Verification items for this drawing (mm, ordinates from the low corner). A direction names the side the tool comes from. Coordinates: 2 decimals unless noted, no trailing zeros. Write each loop counter-clockwise with the first axis right and the second up, starting at its lowest first coordinate (ties: lowest second). Pieces come first, ordered by that corner, then holes. Notation, with made-up numbers: (-30.75, 14) -> (12.25, 14) arc R20 cw to (12.25, 49) -> close; hole circle Ø9 at (29, 80). An arc over 180 degrees is marked (long way). One line per question, with ' | ' between items.
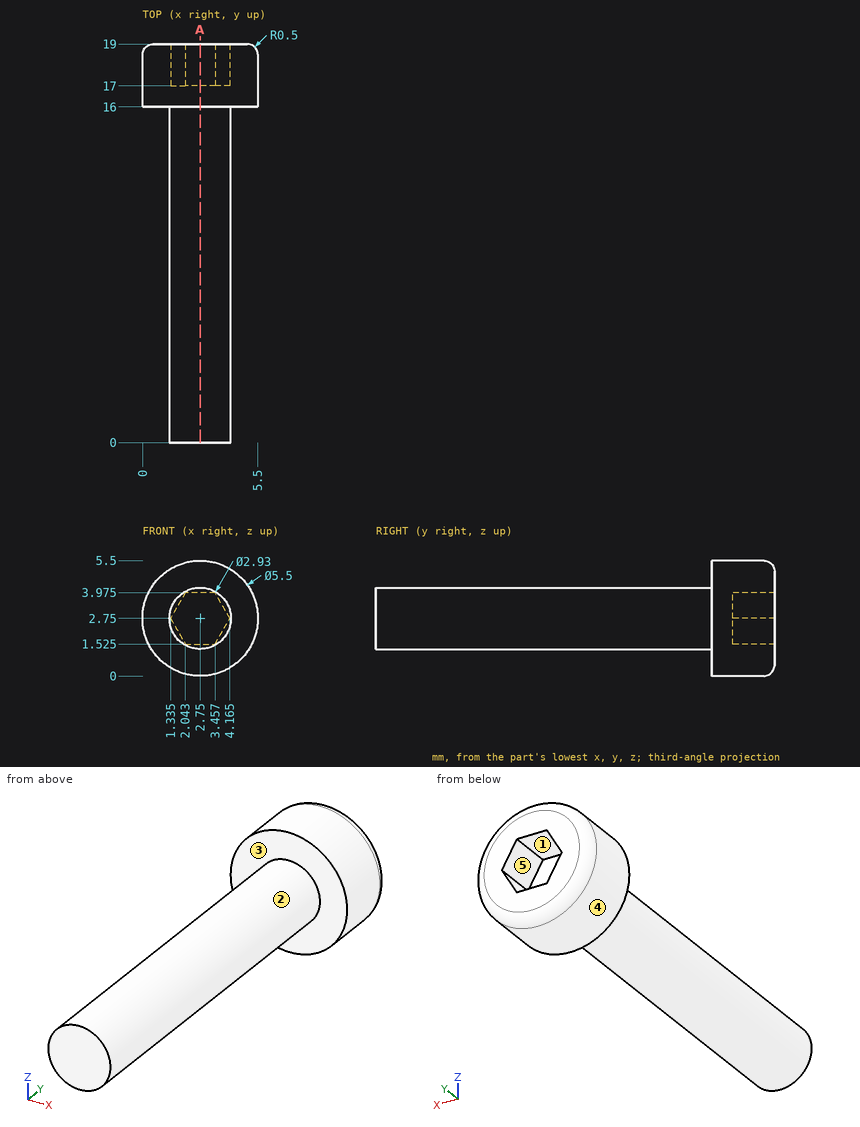
(1) Tool access check on the marked faces 4 and 5. Record the directions out of +Z, -Z, +X, -X, +Y, -Y that give a thin tool (end or side, any length) a straight path to the whole face; none if there is none.
Answers below:
face 4: +Y, -Y | face 5: +Y
(2) Material ranges on line 1 (Y direction, x = 2.9, z = 0.45); line 2 (Y direction, x = 3.5, z = 2.8); line 3 (Z direction, x = 2.7, y = 11) (1 decimal), recorded low to high.
Answers below:
line 1: y = 16 to 19 | line 2: y = 0 to 17 | line 3: z = 1.3 to 4.2
(3) Draft check along X on the marked faces 1, 2 and 3. Enter one of: pulls with the +X half, pulls with the -X half, needs draft (parallel to the pull), parting line crosses it, or undercut.
Answers below:
face 1: undercut | face 2: parting line crosses it | face 3: needs draft
(4) Depth check by flat-ended pin: P1, Ø1, axis at x = 0.5, z = 4.5, coming from the +Y side; P2, Ø1.5, axis at y = 2.5, z = 4.5, coming from the -X side; P3, Ø1.5, axis at y = 16, z = 5, coming from the +X side (1 decimal). Enter the tip coordinate at first touch or a pass-through.
Answers below:
P1: stops at y = 18.99 | P2: stops at x = 1.68 | P3: stops at x = 5.1
(5) Cross-section at A-A (x = 2.75). Record the cut outline in (y, z) (1 decimal).
Answers below:
outline: (0, 1.3) -> (16, 1.3) -> (16, 0) -> (18.5, 0) arc R0.5 ccw to (19, 0.5) -> (19, 1.5) -> (17, 1.5) -> (17, 4) -> (19, 4) -> (19, 5) arc R0.5 ccw to (18.5, 5.5) -> (16, 5.5) -> (16, 4.2) -> (0, 4.2) -> close
